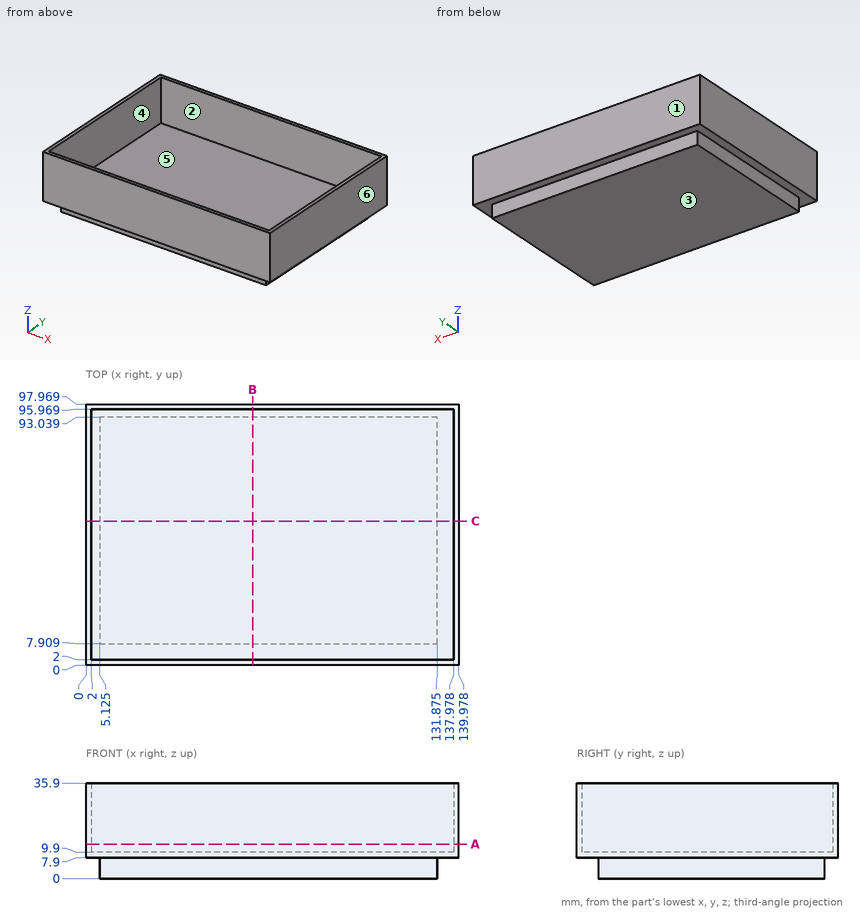
For this review, use the dimensioned drawing (mm, ordinates from the lowest corner) and the shaded views. A direction names the side the tool comes from. Round coordinates to 2 decimals unless told otherwise and drop trailing zeros. Order: outer loops, then holes, each group sorted by start corner. A loop starts at its lowest first (then second) coordinate and runs counter-clockwise, first axis right, second up. Notation, with made-up numbers: (24.25, 31.5) -> (78.25, 31.5) arc R11 cw to (78.25, 39.5) -> close; hole circle Ø5 at (52.25, 87). An arc over 180 degrees is marked (long way). One line per item, written item: value. Start each with the question number.
Q1. Clearance check with flat-ended pins moving along their axes: pin 1 Ø2.5 at (x, z) = (66.5, 2.5) entering from -Y; pin 2 Ø5 at (y, z) = (26, 4) entering from +X (1 decimal); pin 3 Ø5 at (y, z) = (61.5, 5) entering from -X (1 decimal). State where each tip first meets the part, or that it passes through.
Q2. Mouldability with a two-part tool opening along X and no side actions: class the marked faces 3, 4, 5 and 6 as released by +X, released by -X, zero draft, split by the parting line, or undercut.
Q3. Take a section at B-B (x = 62.5). Write out the cut boundary in (y, z).
Q4. Take a section at A-A (z = 13). Write out the cut boundary in (x, y).
Q5. Wall thickness on line 1 (X direction, y = 15, z = 20.5); line 2 (Y direction, x = 119, z = 19); line 3 (Y direction, x = 118.5, z = 5): over which ranges is each line inside the solid? List them lowest first.
Q6. Machinability: for the marked faces 1 and 2, which of the approach directions +Z, -Z, +X, -X, +Y, -Y give a long, thin tool a straight path to every point of the face, cutting with its end or side? Answer none if there is none.
Q7. Take a section at C-C (y = 54). Write out the cut boundary in (x, z) (1 decimal).
Reported:
1. pin 1: stops at y = 7.91
1. pin 2: stops at x = 131.9
1. pin 3: stops at x = 5.1
2. face 3: zero draft
2. face 4: undercut
2. face 5: undercut
2. face 6: released by +X
3. outline: (0, 7.9) -> (7.91, 7.9) -> (7.91, 0) -> (93.04, 0) -> (93.04, 7.9) -> (97.97, 7.9) -> (97.97, 35.9) -> (95.97, 35.9) -> (95.97, 9.9) -> (2, 9.9) -> (2, 35.9) -> (0, 35.9) -> close
4. outline: (0, 0) -> (139.98, 0) -> (139.98, 97.97) -> (0, 97.97) -> close; hole (2, 2) -> (137.98, 2) -> (137.98, 95.97) -> (2, 95.97) -> close
5. line 1: x = 0 to 2, 137.98 to 139.98
5. line 2: y = 0 to 2, 95.97 to 97.97
5. line 3: y = 7.91 to 93.04
6. face 1: +Z, -Z, +X, -X, +Y
6. face 2: +Z
7. outline: (0, 7.9) -> (5.1, 7.9) -> (5.1, 0) -> (131.9, 0) -> (131.9, 7.9) -> (140, 7.9) -> (140, 35.9) -> (138, 35.9) -> (138, 9.9) -> (2, 9.9) -> (2, 35.9) -> (0, 35.9) -> close
